Part model, mm, in its own coordinate system. A direction names the side the tool comes from. Give positions to 0.01 mm unless a question says otherwise; leave off trailing zeros. Order: outer loops, then holes, each group sorted by start corner. A loop starts at its lowest first (then second) coordinate and runs counter-clockwise, first axis right, second up. Notation, with made-up numbers: M 87.25,-18.5 L 104.25,-18.5 A24 cw 104.25,15.5 Z; hole C 23.25,24.5 d7. An arc over 180 degrees is marked long. One line per question, with ' | ' between items.
Autodesk Inventor part; units mm, degrees
ref_plane "YZ Plane" through (0, 0, 0) normal (1, 0, 0) x (0, 1, 0)
ref_plane "XZ Plane" through (0, 0, 0) normal (0, 1, 0) x (-1, 0, 0)
ref_plane "XY Plane" through (0, 0, 0) normal (0, 0, 1) x (1, 0, 0)
sketch "Sketch1" plane through (0, 0, 0) normal (1, 0, 0) x (0, 1, 0)
  line L0 (0, -25) -> (42.2, -25)
  line L1 (3.5, -21.5) -> (45.7, -21.5)
  line L2 (42.2, -25) -> (42.2, -67)
  line L3 (45.7, -21.5) -> (45.7, -70.5)
  line L4 (42.2, -67) -> (3.5, -67)
  line L5 (45.7, -70.5) -> (3.5, -70.5)
  line L6 (3.5, -67) -> (0, -67)
  line L7 (3.5, -21.5) -> (3.5, -5.5)
  line L8 (3.5, -5.5) -> (0, -5.5)
  line L9 (0, -5.5) -> (0, -25)
  line L10 (3.5, -70.5) -> (3.5, -86.5)
  line L11 (3.5, -86.5) -> (0, -86.5)
  line L12 (0, -86.5) -> (0, -67)
  point P0 (0, 0)
  dimension "d3" = 42.2
  dimension "d4" = 42
  dimension "d5" = 3.5
  dimension "d7" = 3.5
  dimension "d19" = 16
  dimension "d20" = 16
extrude "Extrusion1" add sketch "Sketch1" against normal blind 13.5
sketch "Sketch3" plane through (0, 3.5, -5.5) normal (0, 1, 0) x (1, 0, 0)
  circle A0 centre (-6.75, 8.75) radius 2.25
  circle A1 centre (-6.75, 72.25) radius 2.25
  line L0 (0, 16) -> (0, 0)
  line L1 (0, 81) -> (0, 65)
  line L2 (0, 0) -> (-13.5, 0)
  line L3 (0, 81) -> (-13.5, 81)
  point P0 (0, -5.5)
  dimension "d21" = 4.5
  dimension "d22" = 4.5
  dimension "d23" = 6.75
  dimension "d24" = 6.75
  dimension "d25" = 8.75
  dimension "d26" = 8.75
extrude "Extrusion3" cut sketch "Sketch3" against normal through all
fillet "Fillet1" radius 3 2 edges at (-6.75, 45.7, -21.5) (-6.75, 45.7, -70.5)
chamfer "Chamfer1" distance 1.5 angle 45 2 edges at (-6.75, 3.5, -21.5) (-6.75, 3.5, -70.5)
sketch "Sketch5" plane through (0, 42.7, -70.5) normal (0, 0, -1) x (-1, 0, 0)
  circle A0 centre (6.75, -12) radius 3.5
  line L0 (13.5, 3) -> (0, 3)
  line L1 (13.5, 0) -> (13.5, -37.7)
  point P0 (0, -42.7)
  dimension "d44" = 7
  dimension "d45" = 15
  dimension "d51" = 6.75
extrude "Extrusion5" cut sketch "Sketch5" against normal through all
pattern_linear "Rectangular Pattern2" count 2 spacing 15 along (0, -1, 0) of "Extrusion5"
properties part number "Stepper Motor Mount"
1. Slice it at C-C on x = -1.75. Give the cut face in (y, z).
Worked out:
outline: M 0,-86.5 L 3.5,-86.5 L 3.5,-72 L 5,-70.5 L 42.7,-70.5 A3 ccw 45.7,-67.5 L 45.7,-24.5 A3 ccw 42.7,-21.5 L 5,-21.5 L 3.5,-20 L 3.5,-5.5 L 0,-5.5 L 0,-25 L 42.2,-25 L 42.2,-67 L 0,-67 Z
2. Slice it at B-B on z = -77.75. Give the cut face in (x, y), then the cut area to 3 significant figures.
Worked out:
outline: M -13.5,0 L -9,0 L -9,3.5 L -13.5,3.5 Z; M -4.5,0 L 0,0 L 0,3.5 L -4.5,3.5 Z | area: 31.5 mm2
3. Probe L1, parallel to Z at x = -6.75, y = 1.4; L2, parallel to Z at x = -3.5, y = 18; L3, parallel to Y at x = -6.75, z = -69.2. List the from-to ranges inside material, lowest first. Write a range as from..to.
Worked out:
L1: z = -86.5..-80, -75.5..-67, -25..-16.5, -12..-5.5 | L2: z = -70.5..-67, -25..-21.5 | L3: y = 0..12.2, 19.2..27.2, 34.2..45.17
4. Drop flat-ended pins along their axis: pin 1 (7 mm diameter, centred on x = -4, y = 31, fed in from -Z); pin 2 (6 mm diameter, centred on x = -6.75, z = -14.25, fed in from -Y); pin 3 (7 mm diameter, centred on x = -9, y = 30.5, fed in from +Z); pin 4 (4 mm diameter, centred on x = -7, z = -10.5, fed in from +Y). Give the stop position or say it passes through.
Worked out:
pin 1: stops at z = -70.5 | pin 2: stops at y = 0 | pin 3: stops at z = -21.5 | pin 4: stops at y = 3.5
5. Slice it at A-A on y = 15.7. Give the cut face in (x, z).
Worked out:
outline: M -13.5,-70.5 L -10.25,-70.5 L -10.25,-67 L -13.5,-67 Z; M -13.5,-25 L -10.25,-25 L -10.25,-21.5 L -13.5,-21.5 Z; M -3.25,-70.5 L 0,-70.5 L 0,-67 L -3.25,-67 Z; M -3.25,-25 L 0,-25 L 0,-21.5 L -3.25,-21.5 Z
6. Slice it at D-D on y = 8. Give the cut face in (x, z), then the cut area to 3 significant figures.
Worked out:
outline: M -13.5,-70.5 L 0,-70.5 L 0,-67 L -13.5,-67 Z; M -13.5,-25 L 0,-25 L 0,-21.5 L -13.5,-21.5 Z | area: 94.5 mm2
7. Tool access for faces 1 (the flat face through (-7, 3.5, -81)), 2 (the flat face through (-7, 3.5, -11)), 3 (the flat face through (-7, 21, -25)): list every direction of +Z, -Z, +X, -X, +Y, -Y with a clear straight run to the whole face (end or side of a thin tool).
Worked out:
face 1: -Z, +X, -X, +Y | face 2: +Z, +X, -X, +Y | face 3: +X, -X, -Y
8. Mould opens along Y. For faces 4 (the flat face through (-7, 42.2, -46)), 5 (the cylindrical face through (-5.991, 12.283, -68.774)), 6 (the flat face through (-7, 2, -5.5)) say: released by +Y, released by -Y, zero draft, split by the parting line, or undercut.
Worked out:
face 4: released by -Y | face 5: undercut | face 6: zero draft
